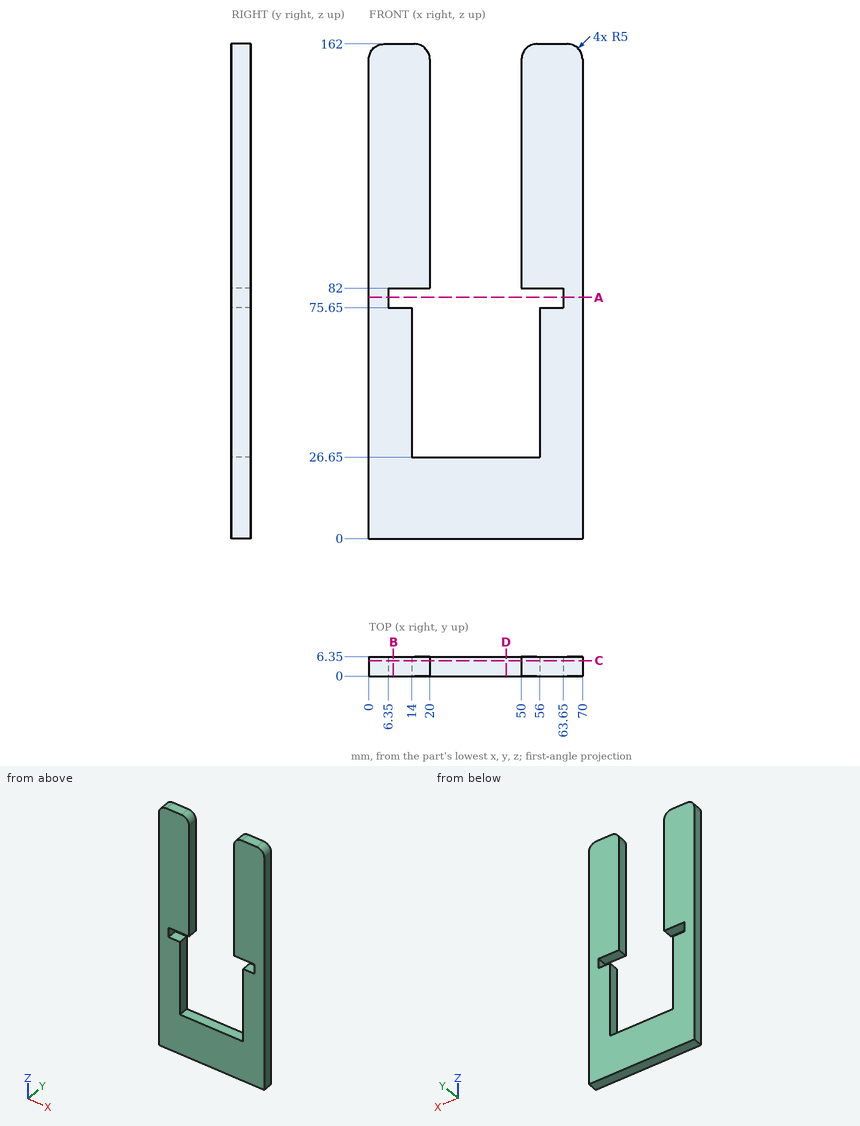
Source: three-view drawing plus pictorial views. Frame: mm from the lowest corner of the part. Give positions to 0.01 mm unless a question says otherwise; leave off trailing zeros. Order: outer loops, then holes, each group sorted by start corner. A loop starts at its lowest first (then second) coordinate and runs counter-clockwise, first axis right, second up. Notation, with made-up numbers: (-14, -0.5) - (-3, -0.5) arc R8 ccw to (-3, 6.5) - close; hole circle Ø9 at (82.25, 24.25). An arc over 180 degrees is marked (long way). Put each result on its own line as item: value.
Item 1: Section query B-B, the plane x = 8. Return loops of the section in (y, z).
Found:
outline: (0, 0) - (6.35, 0) - (6.35, 75.65) - (0, 75.65) - close; (0, 82) - (6.35, 82) - (6.35, 162) - (0, 162) - close
Item 2: Section query D-D, the plane x = 45. Return loops of the section in (y, z).
Found:
outline: (0, 0) - (6.35, 0) - (6.35, 26.65) - (0, 26.65) - close
Item 3: Contact query for flat-ended pins moving along their axis: pin 1 (3 mm diameter, centred on x = 36.5, y = 4, fed in from -Z); pin 2 (3 mm diameter, centred on x = 40, y = 4.5, fed in from +Z). Output: stop coordinate, or through.
Found:
pin 1: stops at z = 0
pin 2: stops at z = 26.65
Item 4: Ray query, L1, parallel to X at y = 2, z = 89.5; L2, parallel to Z at x = 55.5, y = 6; L3, parallel to X at y = 4.25, z = 49.5. Return the intervals inside material, ascending. Write a range as from..to.
Found:
L1: x = 0..20, 50..70
L2: z = 0..26.65, 82..162
L3: x = 0..14, 56..70
Item 5: Section query A-A, the plane z = 79. Return loops of the section in (x, y), then the cut area to 3 significant figures.
Found:
outline: (0, 0) - (6.35, 0) - (6.35, 6.35) - (0, 6.35) - close; (63.65, 0) - (70, 0) - (70, 6.35) - (63.65, 6.35) - close
area: 80.6 mm^2
Item 6: Section query C-C, the plane y = 5. Return loops of the section in (x, z).
Found:
outline: (0, 0) - (70, 0) - (70, 157) arc R5 ccw to (65, 162) - (55, 162) arc R5 ccw to (50, 157) - (50, 82) - (63.65, 82) - (63.65, 75.65) - (56, 75.65) - (56, 26.65) - (14, 26.65) - (14, 75.65) - (6.35, 75.65) - (6.35, 82) - (20, 82) - (20, 157) arc R5 ccw to (15, 162) - (5, 162) arc R5 ccw to (0, 157) - close
